Source: three-view drawing plus pictorial views. Frame: mm from the lowest corner of the part. A direction names the side the tool comes from. Give positions to 0.01 mm unless a question says otherwise; leave off trailing zeros. Write each loop counter-clockwise with the first axis right and the second up, starting at its lowest first coordinate (ties: lowest second). Pieces come first, ordered by that corner, then holes. Notation, with made-up numbers: (74.5, 26) -> (132.5, 26) arc R6 ccw to (132.5, 34) -> close; hole circle Ø6 at (32.5, -20.75). An arc over 180 degrees is marked (long way). Answer in a Markdown table with one row per item. Add a question column.
Item 1: Section query C-C on x = 26. Output: boundary loops of the cut face in (y, z).
Item 2: Access query for the marked faces 1, 2 and 3. Directions: +Z, -Z, +X, -X, +Y, -Y. A direction counts if a zero-diameter tool reaches every point of the face in a straight line with its end or side. Return the directions, or none.
Item 3: Section query B-B on y = 40. Output: boundary loops of the cut face in (x, z).
Item 4: Section query A-A on z = 10. Output: boundary loops of the cut face in (x, y), plus the area to 3 significant figures.
Item 5: Section query D-D on x = 5. Output: boundary loops of the cut face in (y, z).
Item 6: First-contact query: P1, Ø5.5, axis at y = 42, z = 8, coming from the -X side; P2, Ø5, axis at x = 25, y = 9, coming from the +Z side; P3, Ø16.5, axis at x = 12.5, z = 5.5, coming from the +Y side; P4, Ø12, axis at x = 21, z = 14.5, coming from the -Y side. Flat tips, straight axial feed; report the tip coordinate or a pass-through.
Item 7: Material intervals for probe 1 along Y at (x, z) = (25, 10); probe 2 along Y at (x, z) = (7, 5); probe 3 along X at (y, z) = (14.5, 11), sorted ascending. Write a range as from..to.
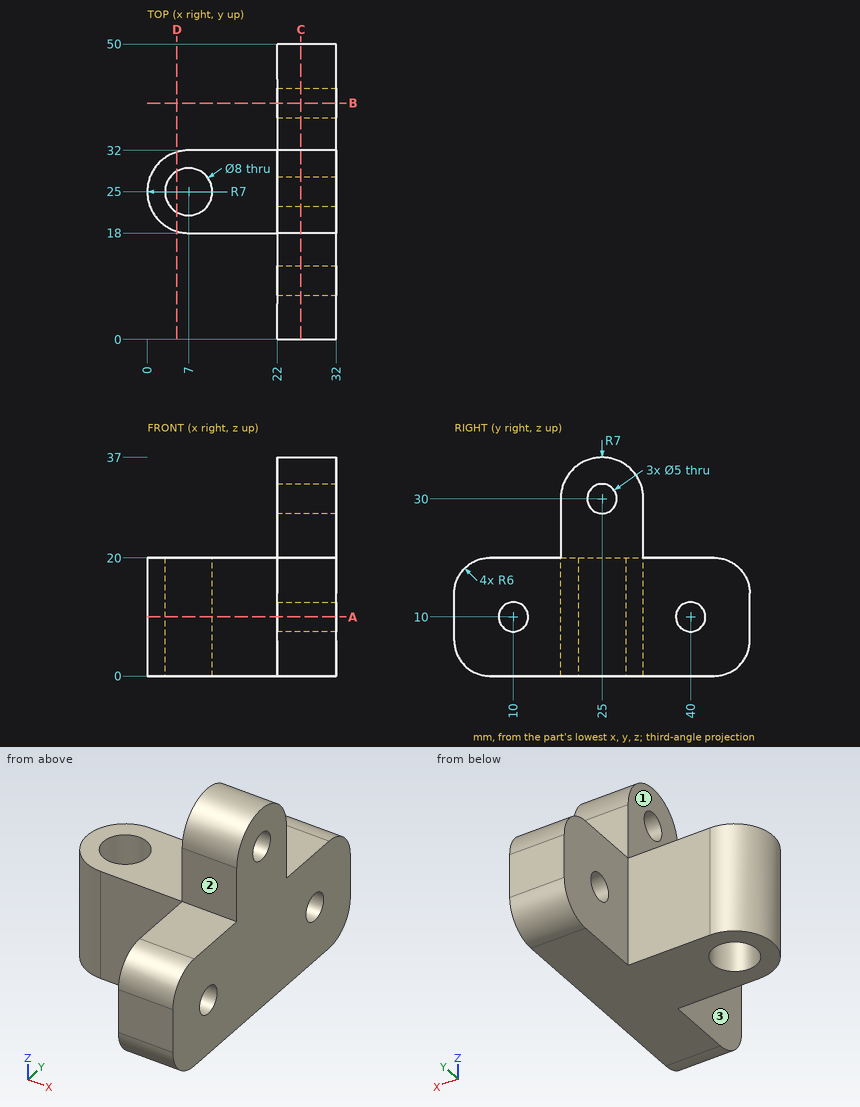
Findings below:
| question | item | result |
|---|---|---|
| 1 | outline | (0, 6) arc R6 ccw to (6, 0) -> (44, 0) arc R6 ccw to (50, 6) -> (50, 14) arc R6 ccw to (44, 20) -> (32, 20) -> (32, 30) arc R7 ccw to (18, 30) -> (18, 20) -> (6, 20) arc R6 ccw to (0, 14) -> close; hole circle Ø5 at (10, 10); hole circle Ø5 at (25, 30); hole circle Ø5 at (40, 10) |
| 2 | face 1 | +Z, -X, +Y, -Y |
| 2 | face 2 | +Z, +X, -X, -Y |
| 2 | face 3 | +Z, -Z, -X, -Y |
| 3 | outline | (22, 0) -> (32, 0) -> (32, 7.5) -> (22, 7.5) -> close; (22, 12.5) -> (32, 12.5) -> (32, 20) -> (22, 20) -> close |
| 4 | outline | (7, 18) -> (22, 18) -> (22, 12.5) -> (32, 12.5) -> (32, 37.5) -> (22, 37.5) -> (22, 32) -> (7, 32) arc R7 ccw to start; (22, 0) -> (32, 0) -> (32, 7.5) -> (22, 7.5) -> close; (22, 42.5) -> (32, 42.5) -> (32, 50) -> (22, 50) -> close; hole circle Ø8 at (7, 25) |
| 4 | area | 637 mm^2 |
| 5 | outline | (18.29, 0) -> (21.54, 0) -> (21.54, 20) -> (18.29, 20) -> close; (28.46, 0) -> (31.71, 0) -> (31.71, 20) -> (28.46, 20) -> close |
| 6 | P1 | stops at x = 22 |
| 6 | P2 | stops at z = 20 |
| 6 | P3 | stops at y = 32 |
| 6 | P4 | stops at y = 0 |
| 7 | probe 1 | y = 0..7.5, 12.5..37.5, 42.5..50 |
| 7 | probe 2 | y = 18..21, 29..32 |
| 7 | probe 3 | x = 22..32 |
